Autodesk Inventor part; units mm, degrees
ref_plane "YZ Plane" through (0, 0, 0) normal (1, 0, 0) x (0, 1, 0)
ref_plane "XZ Plane" through (0, 0, 0) normal (0, 1, 0) x (-1, 0, 0)
ref_plane "XY Plane" through (0, 0, 0) normal (0, 0, 1) x (1, 0, 0)
sketch "Sketch1" plane through (0, 0, 0) normal (0, 1, 0) x (-1, 0, 0)
  circle A0 centre (0, 0) radius 2.0828
  dimension "d4" = 4.1656
extrude "Body" add sketch "Sketch1" along normal blind 7.366
sketch "Sketch2" plane through (0, 0, 0) normal (1, 0, 0) x (0, 1, 0)
  line L0 (7.366, -2.0828) -> (7.366, 2.0828)
  line L1 (7.366, 0) -> (7.366, -3.9624)
  line L2 (7.366, -3.9624) -> (7.747, -3.9624)
  arc A0 (7.747, -3.9624) -> (9.5758, -2.0828) centre (5.5548, 0) ccw
  line L3 (9.5758, -2.0828) -> (9.5758, -1.6764)
  line L4 (9.5758, -1.6764) -> (8.0795, -1.6764)
  line L5 (8.0795, -1.6764) -> (7.4676, 0)
  line L6 (7.4676, 0) -> (7.366, 0)
  point P0 (0, 0)
  dimension "d5" = 3.9624
  dimension "d6" = 0.381
  dimension "d13" = 0.1016
  dimension "d14" = 2.0828
  dimension "d15" = 2.2098
  dimension "d16" = 0
  dimension "d17" = 1.6764
  dimension "d57" = 20.053
revolve "Head" add sketch "Sketch2" angle 360 about axis through (0, 7.4676, 0) along (0, -1, 0)
sketch "Sketch3" plane through (0, 9.5758, 0) normal (0, 1, 0) x (1, 0, 0)
  circle A0 centre (0, 0) radius 1.6764
  line L0 (0.7302, -1.2648) -> (-0.7303, -1.2648) construction
  line L1 (-0.7303, -1.2648) -> (-1.4605, 0) construction
  line L2 (-1.4605, 0) -> (-0.7303, 1.2648) construction
  line L3 (-0.7303, 1.2648) -> (0.7302, 1.2648) construction
  line L4 (0.7302, 1.2648) -> (1.4605, 0) construction
  line L5 (1.4605, 0) -> (0.7302, -1.2648) construction
  circle A1 centre (-0.7303, -1.2648) radius 0.2159
  circle A2 centre (-1.4605, 0) radius 0.2159
  circle A3 centre (-0.7303, 1.2648) radius 0.2159
  circle A4 centre (0.7302, 1.2648) radius 0.2159
  circle A5 centre (1.4605, 0) radius 0.2159
  circle A6 centre (0.7302, -1.2648) radius 0.2159
  circle A7 centre (0, -2.0701) radius 0.8712
  circle A8 centre (0, 2.0701) radius 0.8712
  circle A9 centre (1.7928, -1.0351) radius 0.8712
  circle A10 centre (-1.7928, 1.035) radius 0.8712
  circle A11 centre (1.7928, 1.035) radius 0.8712
  circle A12 centre (-1.7928, -1.0351) radius 0.8712
  circle A13 centre (0, 0) radius 1.8188
  point P0 (0, 0)
  point P1 (0, 0)
  point P2 (0.9413, 1.2192)
  point P3 (1.5265, 0.2056)
  point P4 (1.5265, -0.2056)
  point P5 (0.9413, -1.2192)
  point P6 (0.5852, -1.4248)
  point P7 (-0.5852, -1.4248)
  point P8 (-0.9413, -1.2192)
  point P9 (-1.5265, -0.2056)
  point P10 (-1.5265, 0.2056)
  point P11 (-0.9413, 1.2192)
  point P12 (-0.5852, 1.4248)
  point P13 (0.5852, 1.4248)
  dimension "d58" = 2.921
  dimension "d59" = 4.1402
  dimension "d62" = 120
extrude "Hex" add sketch "Sketch3" against normal blind 1.778 contours A5 A11 A0 | A0 A11 A13 A9 | A0 A9 A5 | A11 A0 | A0 A11 A13 | A9 A13 A0 | A0 A9 | A11 A4 A0 | A0 A8 A13 A11 | A9 A13 A7 A0 | A0 A6 A9 | A4 A8 A0 | A0 A7 A6 | A8 A0 | A7 A0 | A0 A8 A13 | A7 A13 A0 | A3 A0 A8 | A7 A0 A1 | A0 A10 A13 A8 | A7 A13 A12 A0 | A3 A10 A0 | A0 A12 A1 | A10 A0 A13 | A13 A12 A0 | A10 A0 | A0 A12 | A10 A0 A12 A13 | A10 A2 A0 | A0 A2 A12
sketch "Sketch4" plane through (0, 0, 0) normal (0, 0, 1) x (1, 0, 0)
  line L0 (-0.7364, 8.6358) -> (-1.6764, 9.5758)
  line L1 (0, 9.5758) -> (-0.7364, 8.6358)
  line L2 (0, -10.602) -> (0, 63.6118)
  line L3 (-1.5265, 9.5758) -> (-1.5265, 8.0298)
  line L4 (-1.5265, 9.5758) -> (-1.5265, 9.5758)
  line L5 (-1.5265, 9.5758) -> (-1.5265, 8.0298)
  line L6 (-1.6764, 9.5758) -> (-1.5265, 9.5758)
  line L7 (-1.6764, 9.5758) -> (0, 9.5758)
  point P0 (0, 0)
  point P1 (-1.6764, 8.0795)
  dimension "d29" = 1.6764
revolve "Head Chamfer" cut sketch "Sketch4" angle 360 about axis through (0, -10, 0) along (0, 1, 0)
sketch "Sketch5" plane through (0, 0, 0) normal (1, 0, 0) x (0, 1, 0)
  line L0 (0, -2.0828) -> (7.366, -2.0828)
  line L1 (7.366, 3.9624) -> (7.366, -3.9624)
  line L2 (7.366, -2.0828) -> (7.366, 2.0828)
  line L3 (0.0745, -2.0828) -> (-0.2261, -2.6035)
  line L4 (-0.2261, -2.6035) -> (-0.3253, -2.6035)
  line L5 (-0.3253, -2.6035) -> (-0.626, -2.0828)
  line L6 (0.0686, -2.6035) -> (-0.7252, -2.6035) construction
  line L7 (-0.626, -2.0828) -> (0.0745, -2.0828)
  line L8 (0, -2.0828) -> (7.366, -2.0828)
  point P0 (0, 0)
  dimension "d31" = 30
  dimension "d32" = 60
  dimension "a" = 0.0992
  dimension "d46" = 0.7937
  dimension "d54" = 0.0686
  dimension "d55" = 0.5207
  dimension "d56" = 0.0992
feature "Thread" [suppressed]
sketch "Sketch6" plane through (0, 0, 0) normal (0, 0, 1) x (1, 0, 0)
  line L0 (0, 0) -> (-1.4859, 0)
  line L1 (2.0828, 0) -> (-2.0828, 0)
  line L2 (-1.4859, 0) -> (-2.4948, 1.0089)
  line L3 (-2.4948, 1.0089) -> (-2.9651, -1.2188)
  line L4 (-2.9651, -1.2188) -> (-1.4859, -1.2188)
  line L5 (-2.0828, 0) -> (-2.0828, 7.366)
  line L6 (-1.4859, -1.2188) -> (-1.4859, 0)
  line L7 (0, -11.613) -> (0, 61.146)
  point P0 (-2.0828, 0.5969)
  dimension "d49" = 1.4859
  dimension "d50" = 135
revolve "Tapered End" cut sketch "Sketch6" angle 360 about axis through (0, -10, 0) along (0, 1, 0)
sketch "Sketch8" plane through (0, 0, 0) normal (0, 0, 1) x (1, 0, 0)
  line L0 (-3.9624, 7.366) -> (3.9624, 7.366)
  line L1 (0, 7.366) -> (2.286, 7.366)
  line L2 (2.286, 7.366) -> (2.286, 5.08)
  line L3 (2.286, 5.08) -> (0, 5.08)
  line L4 (0, 5.08) -> (0, 7.366)
  point P0 (0, 0)
  dimension "d69" = 2.286
  dimension "d70" = 2.286
revolve "Shoulder" add sketch "Sketch8" angle 360 about axis through (0, 5.08, 0) along (0, 1, 0)
equation "\"d56\" = a"
equation "\"ShoulderLength\" = 2.286"
properties part number "Shoulder Screw 8-32 Shoulder 0.090 Length 0.290" material "VEX Steel"
Can you work these out from the model? Positions are in its coordinate system, mm. A direction names the side the tool comes from. Coordinates: 2 decimals unless noted, no trailing zeros. Loops run counter-clockwise (first coordinate to the right, second up) from the corner with the lowest first, then second, coordinate; pieces in that order, holes last. Notation, with made-up numbers: (-6, 26.5) - (36, 26.5) arc R32 cw to (36, 52.5) - close; hole circle Ø2 at (-2.5, -4.5). An arc over 180 degrees is marked (long way). Answer as CSV lines item,"result". Start each with the question number.
1) Thinking about a two-plate mould opening in X: for faces 3 (the cylindrical face through (-1.043, 8.513, -0.592)), 4 (the cylindrical face through (-3.93, 7.56, 0.52)), 5 (the flat face through (0, 0, 0)), 6 (the conical face through (0.102, 7.506, 0.023)), which applies, pulls with the +X half, pulls with the -X half, needs draft (parallel to the pull), parting line crosses it, or undercut?
2) I need wall thicknesses on line 1 (Z direction, x = 0, y = 3); line 2 (Z direction, x = -0.75, y = 9); line 3 (Y direction, x = 2, z = -2). Which ranges of each line are inside material? Lowest first, please. Write a range as from..to.
3) Suppose I cut it at A-A (y = 3.5). Please give me the cut outline in (x, z), plus the area to 3 significant figures.
4) Which directions (+Z, -Z, +X, -X, +Y, -Y) give clear straight access to the entire face, cutting with the end or side of a thin tool? Please do faces 1 (the cylindrical face through (-0.5, 6.21, -2.23)), 2 (the cylindrical face through (1.034, 8.513, -0.607)).
5) Suppose I cut it at B-B (y = 6.25). Please give me the cut outline in (x, z), plus the area to 3 significant figures.
6) For pin 1 (1.5 mm diameter, centred on y = 8.5, z = -3, fed in from +X); pin 2 (1 mm diameter, centred on x = -2, y = 2, fed in from +Z) (3 decimals); pin 3 (1.5 mm diameter, centred on y = 6, z = 1, fed in from -X), each with a flat end and sliding along its axis, tell me the tip position at first contact or that it passes through.
Check result:
1,face 3,"undercut"
1,face 4,"parting line crosses it"
1,face 5,"needs draft"
1,face 6,"undercut"
2,line 1,"z = -2.08..2.08"
2,line 2,"z = -2.84..-1.48, 1.48..2.84"
2,line 3,"y = 7.37..9.09"
3,outline,"circle Ø4.17 at (0, 0)"
3,area,"13.6 mm²"
4,face 1,"-Y"
4,face 2,"+Y"
5,outline,"circle Ø4.57 at (0, 0)"
5,area,"16.4 mm²"
6,pin 1,"stops at x = 2.93"
6,pin 2,"stops at z = 1.445"
6,pin 3,"stops at x = -2.27"
